The model under review builds one solid part; all positions refer to its coordinate system, in mm. Face numbers are marked on the shaded views. A direction names the side the tool comes from. Give positions to 0.01 mm unless a question says otherwise; leave off trailing zeros. Write each loop counter-clockwise with the first axis right and the second up, starting at its lowest first coordinate (ties: lowest second). Pieces come first, ordered by that corner, then holes. Notation, with made-up numbers: (42.5, -22.75) - (77.5, -22.75) arc R29 ccw to (77.5, 9.25) - close; hole circle Ø3 at (-39, -33.5). An arc over 180 degrees is marked (long way). Write item = value, one per line.
```python
from build123d import *

# Parameters (mm, degrees)
SKETCH2_R             = 4.5
BOSS_EXTRUDE1_DEPTH   = 30
BOSS_EXTRUDE1_2_DEPTH = 30
BOSS_EXTRUDE1_3_DEPTH = 30
BOSS_EXTRUDE1_4_DEPTH = 30
BOSS_EXTRUDE1_5_DEPTH = 30
SKETCH3_R             = 29.35
SKETCH3_R_2           = 20.65
BOSS_EXTRUDE2_DEPTH   = 3
SKETCH4_R             = 4.5
BOSS_EXTRUDE3_DEPTH   = 2
SKETCH5_R             = 4.5
SKETCH5_R_2           = 4.275
CUT_EXTRUDE1_DEPTH    = 13
CHAMFER1_SIZE         = 1
SKETCH6_R             = 4.55
BOSS_EXTRUDE4_DEPTH   = 17.5


with BuildPart() as part:
    # Sketch2 → Boss-Extrude1 (new body)
    with BuildSketch(Plane(origin=(0, 0, -6.013631981), x_dir=(-1, 0, 0), z_dir=(0, 0, -1))):
        with Locations((-11.73472812, -13.580511576)):
            Circle(SKETCH2_R)
    extrude(amount=BOSS_EXTRUDE1_DEPTH)



with BuildPart() as body_2:
    # Sketch2 → Boss-Extrude1 2 (new body)
    with BuildSketch(Plane(origin=(0, 0, -6.013631981), x_dir=(-1, 0, 0), z_dir=(0, 0, -1))):
        with Locations((4.847454424, -37.844888326)):
            Circle(SKETCH2_R)
    extrude(amount=BOSS_EXTRUDE1_2_DEPTH)


with BuildPart() as body_3:
    # Sketch2 → Boss-Extrude1 3 (new body)
    with BuildSketch(Plane(origin=(0, 0, -6.013631981), x_dir=(-1, 0, 0), z_dir=(0, 0, -1))):
        with Locations((-13.105162988, -61.113585864)):
            Circle(SKETCH2_R)
    extrude(amount=BOSS_EXTRUDE1_3_DEPTH)


with BuildPart() as body_4:
    # Sketch2 → Boss-Extrude1 4 (new body)
    with BuildSketch(Plane(origin=(0, 0, -6.013631981), x_dir=(-1, 0, 0), z_dir=(0, 0, -1))):
        with Locations((-40.78267328, -51.230055065)):
            Circle(SKETCH2_R)
    extrude(amount=BOSS_EXTRUDE1_4_DEPTH)


with BuildPart() as body_5:
    # Sketch2 → Boss-Extrude1 5 (new body)
    with BuildSketch(Plane(origin=(0, 0, -6.013631981), x_dir=(-1, 0, 0), z_dir=(0, 0, -1))):
        with Locations((-39.935697953, -21.852999565)):
            Circle(SKETCH2_R)
    extrude(amount=BOSS_EXTRUDE1_5_DEPTH)


with BuildPart() as part_1:
    add(part.part)

    add(body_2.part)  # Boss-Extrude2 merges body 2

    add(body_3.part)  # Boss-Extrude2 merges body 3

    add(body_4.part)  # Boss-Extrude2 merges body 4

    add(body_5.part)  # Boss-Extrude2 merges body 5
    # Sketch3 → Boss-Extrude2 (add)
    with BuildSketch(Plane.XY.offset(-6.013631981)):
        with Locations((20.142161583, -37.124408079)):
            Circle(SKETCH3_R)
        with Locations((20.142161583, -37.124408079)):
            Circle(SKETCH3_R_2, mode=Mode.SUBTRACT)
    extrude(amount=BOSS_EXTRUDE2_DEPTH)

    # Sketch4 → Boss-Extrude3 (add)
    with BuildSketch(Plane(origin=(0, 0, -36.013631981), x_dir=(-1, 0, 0), z_dir=(0, 0, -1))):
        with Locations((4.847454424, -37.844888326)):
            Circle(SKETCH4_R)
        with Locations((-11.73472812, -13.580511576)):
            Circle(SKETCH4_R)
        with Locations((-39.935697953, -21.852999565)):
            Circle(SKETCH4_R)
        with Locations((-40.78267328, -51.230055065)):
            Circle(SKETCH4_R)
        with Locations((-13.105162988, -61.113585864)):
            Circle(SKETCH4_R)
    extrude(amount=BOSS_EXTRUDE3_DEPTH)

    # Sketch5 → Cut-Extrude1 (cut)
    with BuildSketch(Plane(origin=(0, 0, -38.013631981), x_dir=(-1, 0, 0), z_dir=(0, 0, -1))):
        with Locations((-13.105162988, -61.113585864)):
            Circle(SKETCH5_R)
        with Locations((-13.105162988, -61.113585864)):
            Circle(SKETCH5_R_2, mode=Mode.SUBTRACT)
        with Locations((-40.78267328, -51.230055065)):
            Circle(SKETCH5_R)
        with Locations((-40.78267328, -51.230055065)):
            Circle(SKETCH5_R_2, mode=Mode.SUBTRACT)
        with Locations((-39.935697953, -21.852999565)):
            Circle(SKETCH5_R)
        with Locations((-39.935697953, -21.852999565)):
            Circle(SKETCH5_R_2, mode=Mode.SUBTRACT)
        with Locations((-11.73472812, -13.580511576)):
            Circle(SKETCH5_R)
        with Locations((-11.73472812, -13.580511576)):
            Circle(SKETCH5_R_2, mode=Mode.SUBTRACT)
        with Locations((4.847454424, -37.844888326)):
            Circle(SKETCH5_R)
        with Locations((4.847454424, -37.844888326)):
            Circle(SKETCH5_R_2, mode=Mode.SUBTRACT)
    extrude(amount=-CUT_EXTRUDE1_DEPTH, mode=Mode.SUBTRACT)

    # Chamfer1
    chamfer1_edges = [part_1.edges().sort_by_distance(p)[0] for p in [
        (17.380162988, -61.113585864, -38.013631981),
        (45.05767328, -51.230055065, -38.013631981),
        (44.210697953, -21.852999565, -38.013631981),
        (16.00972812, -13.580511576, -38.013631981),
        (-0.572454424, -37.844888326, -38.013631981),
    ]]
    chamfer(chamfer1_edges, length=CHAMFER1_SIZE)

    # Sketch6 → Boss-Extrude4 (add)
    with BuildSketch(Plane(origin=(0, 0, -25.013631981), x_dir=(-1, 0, 0), z_dir=(0, 0, -1))):
        with Locations((-13.105162988, -61.113585864)):
            Circle(SKETCH6_R)
    extrude(amount=-BOSS_EXTRUDE4_DEPTH)


solid = part_1.part
```
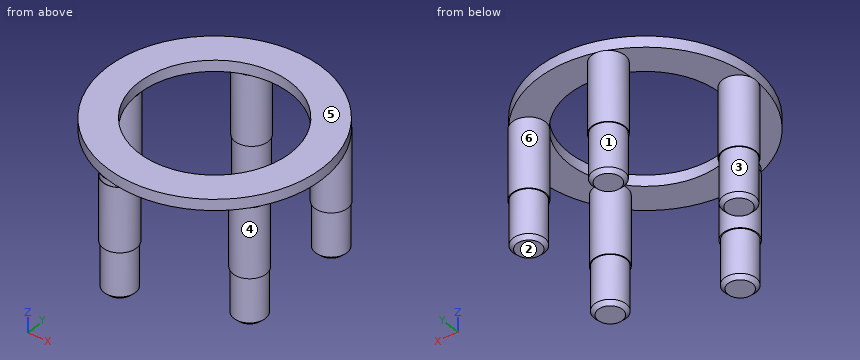
1. For line 1 (Z direction, x = 45.5, y = -37.5); line 2 (Y direction, x = 15, z = -26); line 3 (X direction, y = -39, z = -12), list the stretches that pass through material, from the lowest coordinate up. Write a range as from..to.
Findings below:
line_1 = -6.01..-3.01
line_2 = -64.95..-57.28, -16.34..-10.82
line_3 = -9.2..-0.5
2. Insertion check: P1, Ø8.5, axis at x = 29.5, y = -59, coming from the -Z side; P2, Ø1, axis at x = 36, y = -24.5, coming from the +Z side; P3, Ø12, axis at y = -40, z = -22, coming from the +X side; P4, Ø1.5, axis at y = -59, z = -7, coming from the +X side. Each pin has a flat end and moves straight along its axis. Give the tip position at first contact, or say it passes through.
Findings below:
P1 = -6.01
P2 = -3.01
P3 = -0.35
P4 = 17.39
3. Take a section at C-C on z = -11.5. Give the boundary of the cut face in (x, y).
Findings below:
outline = circle Ø9 at (-4.85, -37.84); circle Ø9 at (11.73, -13.58); circle Ø9.1 at (13.11, -61.11); circle Ø9 at (39.94, -21.85); circle Ø9 at (40.78, -51.23)
4. Take a section at D-D on z = -27.5. Give the boundary of the cut face in (x, y) (3 decimals).
Findings below:
outline = circle Ø8.55 at (-4.847, -37.845); circle Ø8.55 at (11.735, -13.581); circle Ø8.55 at (13.105, -61.114); circle Ø8.55 at (39.936, -21.853); circle Ø8.55 at (40.783, -51.23)
5. Take a section at A-A on x = 20.5. Give the boundary of the cut face in (y, z).
Findings below:
outline = (-66.47, -6.01) - (-57.77, -6.01) - (-57.77, -3.01) - (-66.47, -3.01) - close; (-16.48, -6.01) - (-7.78, -6.01) - (-7.78, -3.01) - (-16.48, -3.01) - close
6. Draft analysis for pull direction Y (two halves, no side actions). For the marked faces 3, 4, 5 and 6, state which applies: +Y half, -Y half, draft (parallel to the pull), parting line (faces both ways), or undercut.
Findings below:
face_3 = parting line
face_4 = undercut
face_5 = draft
face_6 = undercut
7. Machinability: for the marked faces 1 and 2, which of the approach directions +Z, -Z, +X, -X, +Y, -Y give a long, thin tool a straight path to every point of the face, cutting with its end or side? Answer none if there is none.
Findings below:
face_1 = -Z
face_2 = -Z, +X, -X, +Y, -Y
8. Take a section at B-B on y = -29. Give the boundary of the cut face in (x, z), and give its area (3 significant figures).
Findings below:
outline = (-8.06, -6.01) - (1.16, -6.01) - (1.16, -3.01) - (-8.06, -3.01) - close; (39.13, -6.01) - (48.35, -6.01) - (48.35, -3.01) - (39.13, -3.01) - close
area = 55.3 mm²
